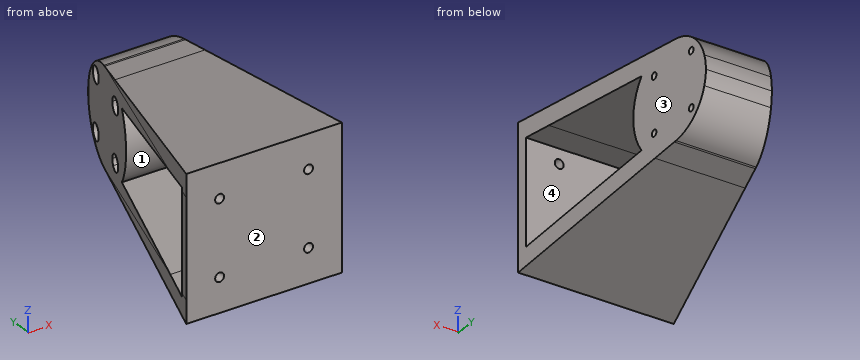
```python
from build123d import *
from build123d import SkipClean  # not in build123d's __all__

# Parameters (mm, degrees)
F1_DEPTH = 43
F2_R     = 1.5
F3_DEPTH = 76.2
F4_REACH = 159.0367669999
F5_R     = 2
F6_DEPTH = 5
F7_START = -10
F2_R_2   = 3.6
F7_DEPTH = 40


with BuildPart() as f1:
    # F0 (on Top) → F1 (new body)
    with BuildSketch(Plane.XY):
        Polygon((17.0276526734, -48.2698833057), (17.0276526734, 72.2301166943), (-12.9723473266, 72.2301166943), (-52.9723473266, -48.2698833057), align=None)
    extrude(amount=F1_DEPTH)

    # F2 (on face) → F3 (cut)
    with BuildSketch(Plane.YZ.offset(17.0276526734)):
        with Locations((63.7509319745, 9.4791847198)):
            Circle(F2_R)
        with Locations((63.7509319745, 33.5208152802)):
            Circle(F2_R)
        with Locations((39.7093014141, 33.5208152802)):
            Circle(F2_R)
        with Locations((39.7093014141, 9.4791847198)):
            Circle(F2_R)
        with BuildLine():
            Line((72.2301166943, 36.6657508881), (72.2301166943, 43))
            Line((72.2301166943, 43), (65.4414258951, 43))
            ThreePointArc((65.4414258951, 43), (69.1264984233, 40.1444603767), (72.2301166943, 36.6657508881))
        make_face()
        with BuildLine():
            Line((72.2301166943, 0), (72.2301166943, 6.3342491119))
            ThreePointArc((72.2301166943, 6.3342491119), (69.1264984233, 2.8555396233), (65.4414258951, 0))
            Line((65.4414258951, 0), (72.2301166943, 0))
        make_face()
        with BuildLine():
            ThreePointArc((31.5312779311, 5.93539552), (26.2301166943, 21.5), (31.5312779311, 37.06460448))
            Line((31.5312779311, 37.06460448), (-28.4524949389, 43))
            Line((-28.4524949389, 43), (-43.2698833057, 43))
            Line((-43.2698833057, 43), (-43.2698833057, 0))
            Line((-43.2698833057, 0), (-28.4524949389, 0))
            Line((-28.4524949389, 0), (31.5312779311, 5.93539552))
        make_face()
        with BuildLine():
            ThreePointArc((72.2301166943, 36.6657508881), (69.1264984233, 40.1444603767), (65.4414258951, 43))
            Line((65.4414258951, 43), (52.7912383465, 43))
            Line((52.7912383465, 43), (53.8472030595, 42.8955122706))
            ThreePointArc((53.8472030595, 42.8955122706), (65.276177069, 38.1959350838), (72.2301166943, 27.9807406984))
            Line((72.2301166943, 27.9807406984), (72.2301166943, 36.6657508881))
        make_face()
        with BuildLine():
            Line((72.2301166943, 6.3342491119), (72.2301166943, 15.0192593016))
            ThreePointArc((72.2301166943, 15.0192593016), (65.276177069, 4.8040649162), (53.8472030595, 0.1044877294))
            Line((53.8472030595, 0.1044877294), (52.7912383465, 0))
            Line((52.7912383465, 0), (65.4414258951, 0))
            ThreePointArc((65.4414258951, 0), (69.1264984233, 2.8555396233), (72.2301166943, 6.3342491119))
        make_face()
    extrude(amount=-F3_DEPTH, mode=Mode.SUBTRACT)

    f4_end = Plane(origin=(-22.9147509124, 42.2786258919, 21.5), x_dir=(-0.3150460979, -0.94907637, 0), z_dir=(-0.94907637, 0.3150460979, 0))
    # F2 (on face) → F4 (join, up to a plane its end follows)
    with BuildSketch(Plane.YZ.offset(17.0276526734)):
        Polygon((-43.2698833057, 0), (-48.2698833057, 0), (-48.2698833057, -1.9609309735), (-43.2698833057, -1.466180874), align=None)
        with BuildLine():
            Line((-48.2698833057, -10), (40.2025293734, -1.2456530036))
            ThreePointArc((40.2025293734, -1.2456530036), (39.0953081378, -0.6497542366), (38.0188074935, 0))
            Line((38.0188074935, 0), (-28.4524949389, 0))
            Line((-28.4524949389, 0), (-43.2698833057, -1.466180874))
            Line((-43.2698833057, -1.466180874), (-48.2698833057, -1.9609309735))
            Line((-48.2698833057, -1.9609309735), (-48.2698833057, -10))
        make_face()
        Polygon((-43.2698833057, 44.466180874), (-48.2698833057, 44.9609309735), (-48.2698833057, 43), (-43.2698833057, 43), align=None)
        with BuildLine():
            ThreePointArc((38.0188074935, 43), (39.0953081378, 43.6497542366), (40.2025293734, 44.2456530036))
            Line((40.2025293734, 44.2456530036), (-48.2698833057, 53))
            Line((-48.2698833057, 53), (-48.2698833057, 44.9609309735))
            Line((-48.2698833057, 44.9609309735), (-43.2698833057, 44.466180874))
            Line((-43.2698833057, 44.466180874), (-28.4524949389, 43))
            Line((-28.4524949389, 43), (38.0188074935, 43))
        make_face()
        with BuildLine():
            Line((51.7301166943, 43), (52.7912383465, 43))
            Line((52.7912383465, 43), (40.2025293734, 44.2456530036))
            ThreePointArc((40.2025293734, 44.2456530036), (39.0953081378, 43.6497542366), (38.0188074935, 43))
            Line((38.0188074935, 43), (51.7301166943, 43))
        make_face()
        with BuildLine():
            Line((52.7912383465, 0), (51.7301166943, 0))
            Line((51.7301166943, 0), (38.0188074935, 0))
            ThreePointArc((38.0188074935, 0), (39.0953081378, -0.6497542366), (40.2025293734, -1.2456530036))
            Line((40.2025293734, -1.2456530036), (52.7912383465, 0))
        make_face()
        with BuildLine():
            ThreePointArc((73.2301166943, 21.5), (72.9786460552, 24.7787192622), (72.2301166943, 27.9807406984))
            Line((72.2301166943, 27.9807406984), (72.2301166943, 15.0192593016))
            ThreePointArc((72.2301166943, 15.0192593016), (72.9786460552, 18.2212807378), (73.2301166943, 21.5))
        make_face()
    f4_long = extrude(amount=-F4_REACH, mode=Mode.PRIVATE)
    add(split(f4_long, bisect_by=f4_end, keep=Keep.BOTTOM, mode=Mode.PRIVATE))

    # F5 (on face) → F6 (cut)
    with BuildSketch(Plane.XZ.offset(48.2698833057)):
        with Locations((2.0276526734, 5)):
            Circle(F5_R)
        with Locations((2.0276526734, 38)):
            Circle(F5_R)
        with Locations((-37.9723473266, 38)):
            Circle(F5_R)
        with Locations((-37.9723473266, 5)):
            Circle(F5_R)
    extrude(amount=-F6_DEPTH, mode=Mode.SUBTRACT)

    # F2 (on face) → F7 (cut)
    with BuildSketch(Plane.YZ.offset(17.0276526734).offset(F7_START)):
        with Locations((63.7509319745, 33.5208152802)):
            Circle(F2_R_2)
        with Locations((63.7509319745, 33.5208152802)):
            Circle(F2_R, mode=Mode.SUBTRACT)
        with BuildLine():
            Line((42.3226328457, 35.9967996963), (37.6318949116, 36.4609483083))
            ThreePointArc((37.6318949116, 36.4609483083), (38.0538050247, 30.3240463325), (43.3093014141, 33.5208152802))
            ThreePointArc((43.3093014141, 33.5208152802), (43.0535496969, 34.8534830644), (42.3226328457, 35.9967996963))
        make_face()
        with Locations((39.7093014141, 33.5208152802)):
            Circle(F2_R, mode=Mode.SUBTRACT)
        with BuildLine():
            ThreePointArc((42.3226328457, 35.9967996963), (40.0637902939, 37.1033196604), (37.6318949116, 36.4609483083))
            Line((37.6318949116, 36.4609483083), (42.3226328457, 35.9967996963))
        make_face()
        with BuildLine():
            Line((42.3226328457, 7.0032003037), (37.6318949116, 6.5390516917))
            ThreePointArc((37.6318949116, 6.5390516917), (40.0637902939, 5.8966803396), (42.3226328457, 7.0032003037))
        make_face()
        with BuildLine():
            ThreePointArc((43.3093014141, 9.4791847198), (38.0538050247, 12.6759536675), (37.6318949116, 6.5390516917))
            Line((37.6318949116, 6.5390516917), (42.3226328457, 7.0032003037))
            ThreePointArc((42.3226328457, 7.0032003037), (43.0535496969, 8.1465169356), (43.3093014141, 9.4791847198))
        make_face()
        with Locations((39.7093014141, 9.4791847198)):
            Circle(F2_R, mode=Mode.SUBTRACT)
        with Locations((63.7509319745, 9.4791847198)):
            Circle(F2_R_2)
        with Locations((63.7509319745, 9.4791847198)):
            Circle(F2_R, mode=Mode.SUBTRACT)
    extrude(amount=-F7_DEPTH, mode=Mode.SUBTRACT)


solid = f1.part
```
Work out the finished part from the listing and answer in its coordinate system (mm). Face numbers are marked on the shaded views. A direction names the side the tool comes from. Give positions to 0.01 mm unless a question says otherwise; leave off trailing zeros. Loops run counter-clockwise (first coordinate to the right, second up) from the corner with the lowest first, then second, coordinate; pieces in that order, holes last. Notation, with made-up numbers: (26.5, 29) -> (33.5, 29) arc R20 ccw to (33.5, 54) -> close; hole circle Ø8 at (51.5, 43.25). An arc over 180 degrees is marked (long way). Put each result on its own line as item: value. Start each with the question number.
Item 1: The part is cut by section A-A (x = 10). Give the vertices of the cut face in (y, z).
Item 2: The part is cut by section D-D (x = -21). Give the vertices of the cut face in (y, z), then the cut area to 3 significant figures.
Item 3: Which of the six approach directions +Z, -Z, +X, -X, +Y, -Y give full straight-line access (tool end or side, diameter ignored) to the marked faces 3 and 4?
Item 4: Find the intervals of material crossed by L1, parallel to Z at x = -19.5, y = 41; L2, parallel to Y at x = -46, z = 41.5; L3, parallel to Y at x = 11.5, z = 10, in increasing order. Write a range as [from, to].
Item 5: Each of these flat-tipped pins is pushed along its axis until it touches: P1, Ø4.5, axis at x = -37.97, z = 5, coming from the +Y side; P2, Ø2, axis at y = 40, z = 32, coming from the -X side; P3, Ø1, axis at y = 50, z = 20.5, coming from the -X side. Where does it stop, or does it pass through?
Item 6: The mould has two halves that part along Z. Classify the marked faces 1 and 2: released by +Z, released by -Z, zero draft, split by the parting line, or undercut.
Item 7: The part is cut by section C-C (z = 19). Give the vertices of the cut face in (x, y), then the cut area to 3 significant figures.
Item 8: The part is cut by section B-B (y = -11). Give the vertices of the cut face in (x, z).
Answers below:
1. outline: (-48.27, -10) -> (53.85, 0.1) arc R21.5 ccw to (53.85, 42.9) -> (-48.27, 53) -> close; hole (-43.27, -1.47) -> (31.53, 5.94) arc R25.5 cw to (31.53, 37.06) -> (-43.27, 44.47) -> close; hole circle Ø3 at (39.71, 9.48); hole circle Ø3 at (39.71, 33.52); hole circle Ø3 at (63.75, 9.48); hole circle Ø3 at (63.75, 33.52)
2. outline: (-48.27, -10) -> (48.05, -0.47) -> (48.05, 43.47) -> (-48.27, 53) -> close; hole (-43.27, -1.47) -> (31.53, 5.94) arc R25.5 cw to (31.53, 37.06) -> (-43.27, 44.47) -> close; hole circle Ø7.2 at (39.71, 9.48); hole circle Ø7.2 at (39.71, 33.52)
2. area: 2,300 mm2
3. face 3: +Z, -Z, +X, +Y, -Y
3. face 4: +X, -X
4. L1: [-1.17, 6.12], [12.84, 30.16], [36.88, 44.17]
4. L2: [-48.27, -43.27]
4. L3: [-48.27, -43.27], [28.97, 38.3], [41.12, 62.34], [65.16, 69.9]
5. P1: y = -43.27
5. P2: x = 7.03
5. P3: x = -20.52
6. face 1: undercut
6. face 2: zero draft
7. outline: (-52.97, -48.27) -> (17.03, -48.27) -> (17.03, -43.27) -> (-51.31, -43.27) -> close; (-28.2, 26.35) -> (17.03, 26.35) -> (17.03, 73.08) -> (-12.69, 73.08) -> close
7. area: 2,100 mm2
8. outline: (-40.6, -6.31) -> (17.03, -6.31) -> (17.03, 1.73) -> (-40.6, 1.73) -> close; (-40.6, 41.27) -> (17.03, 41.27) -> (17.03, 49.31) -> (-40.6, 49.31) -> close
